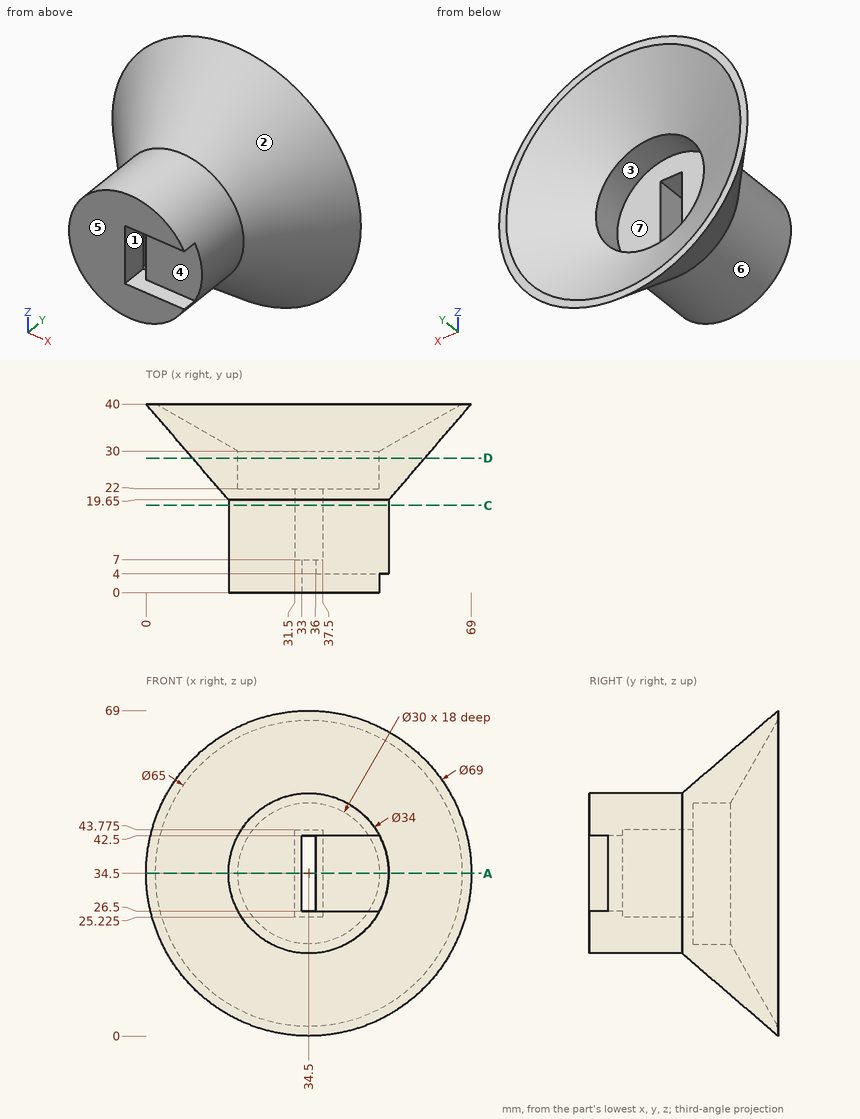
The drawing under review shows one solid part. Ordinate dimensions are in mm from its lowest x, y, z. A direction names the side the tool comes from. Coordinates: 2 decimals unless noted, no trailing zeros. Write each loop counter-clockwise with the first axis right and the second up, starting at its lowest first coordinate (ties: lowest second). Pieces come first, ordered by that corner, then holes.
1) Add section A-A (z = 34.5). Write out the cut boundary in (x, y), plus the area to 3 significant figures.
2) Add section D-D (y = 28.5). Write out the cut boundary in (x, z).
3) To check wall thickness, follow L1, parallel to Y at x = 35, z = 20; L2, parallel to Y at x = 46.5, z = 39; L3, parallel to Z at x = 34, y = 25 (1 decimal). State the ranges of each line that lie inside material, in increasing order.
4) Machinability: for the marked faces 1, 2, 3 and 4, which of the approach directions +Z, -Z, +X, -X, +Y, -Y give a long, thin tool a straight path to every point of the face, cutting with its end or side? Answer none if there is none.
5) Add section C-C (y = 18.5). Write out the cut boundary in (x, z) (1 decimal).
6) Mouldability with a two-part tool opening along Z and no side actions: class the marked faces 5, 6 and 7 as +Z half, -Z half, draft (parallel to the pull), parting line (faces both ways), or undercut.
7) Insertion check: pin 1 (2 mm diameter, centred on x = 56.5, y = 32.5, fed in from +Z) (1 decimal); pin 2 (15 mm diameter, centred on x = 40, z = 29.5, fed in from +Y); pin 3 (2 mm diameter, centred on x = 41.5, z = 34.5, fed in from -Y). Each pin has a flat end and moves straight along its axis. Give the tip position at first contact, or say it passes through.
Check result:
1. outline: (0, 40) - (17.5, 19.65) - (17.5, 0) - (33, 0) - (33, 7) - (31.5, 7) - (31.5, 22) - (19.5, 22) - (19.5, 30) - (2, 40) - close; (36, 4) - (51.5, 4) - (51.5, 19.65) - (69, 40) - (67, 40) - (49.5, 30) - (49.5, 22) - (37.5, 22) - (37.5, 7) - (36, 7) - close
1. area: 828 mm2
2. outline: circle Ø49.22 at (34.5, 34.5); hole circle Ø30 at (34.5, 34.5)
3. L1: y = 0 to 22
3. L2: y = 4 to 22
3. L3: z = 12.9 to 19.5, 49.5 to 56.1
4. face 1: +Y, -Y
4. face 2: -Y
4. face 3: +Y
4. face 4: +X, -Y
5. outline: circle Ø34 at (34.5, 34.5); hole (31.5, 25.2) - (37.5, 25.2) - (37.5, 43.8) - (31.5, 43.8) - close
6. face 5: draft
6. face 6: parting line
6. face 7: undercut
7. pin 1: stops at z = 53.7
7. pin 2: stops at y = 22
7. pin 3: stops at y = 4
